```python
from build123d import *

# Parameters (mm, degrees)
EXTRUDE_1_DEPTH          = 3
EXTRUDE_2_DEPTH          = 287
SKETCH_4_W               = 21.736589458
SKETCH_4_H               = 200
CUT_EXTRUDE_1_DEPTH      = 43
SKETCH_5_W               = 23.415155123
SKETCH_5_H               = 200
CUT_EXTRUDE_2_DEPTH      = 43
CUT_EXTRUDE_3_DEPTH      = 259.263552403
HOLE_WIZARD_1_AT_2_COUNT = 2
HOLE_WIZARD_1_AT_2_PITCH = 31.622776602
HOLE_WIZARD_1_AT_3_COUNT = 2
HOLE_WIZARD_1_AT_3_PITCH = 10
HOLE_WIZARD_1_AT_4_COUNT = 2
HOLE_WIZARD_1_AT_4_PITCH = 242.860042
HOLE_WIZARD_1_AT_5_COUNT = 2
HOLE_WIZARD_1_AT_5_PITCH = 241
HOLE_WIZARD_1_AT_6_COUNT = 2
HOLE_WIZARD_1_AT_6_PITCH = 232.939906414
HOLE_WIZARD_1_AT_7_COUNT = 2
HOLE_WIZARD_1_AT_7_PITCH = 231
HOLE_WIZARD_1_AT_8_COUNT = 2
HOLE_WIZARD_1_AT_8_PITCH = 30
SKETCH_10_W              = 190.5
SKETCH_10_H              = 70
CUT_EXTRUDE_4_DEPTH      = 2
SKETCH_11_W              = 190.5
SKETCH_11_H              = 60
CUT_EXTRUDE_5_DEPTH      = 1


with BuildPart() as part:
    # 草图1 → 凸台-拉伸1 (new body)
    with BuildSketch(Plane.XY):
        Polygon((-143.25, 30), (-143.25, 70), (-105.25, 70), (-105.25, 65), (-100.25, 65), (-100.25, 70), (100.75, 70), (100.75, 65), (105.75, 65), (105.75, 70), (143.75, 70), (143.75, 30), (135.75, 30), (135.75, -30), (143.75, -30), (143.75, -70), (105.75, -70), (105.75, -65), (100.75, -65), (100.75, -70), (-100.25, -70), (-100.25, -65), (-105.25, -65), (-105.25, -70), (-143.25, -70), (-143.25, -30), (-135.25, -30), (-135.25, 30), align=None)
    extrude(amount=EXTRUDE_1_DEPTH)

    # 草图2 → 凸台-拉伸2 (add)
    with BuildSketch(Plane.ZY.offset(143.25)):
        with BuildLine():
            Line((0, 70), (0, 30))
            Line((0, 30), (-3, 33))
            Line((-3, 33), (-3, 70))
            ThreePointArc((-3, 70), (6.665476221, 93.334523779), (30, 103))
            Line((30, 103), (47, 103))
            Line((47, 103), (50, 100))
            Line((50, 100), (45, 90))
            Line((45, 90), (60, 90))
            Line((60, 90), (60, 87))
            Line((60, 87), (41, 87))
            Line((41, 87), (47, 100))
            Line((47, 100), (30, 100))
            ThreePointArc((30, 100), (8.786796564, 91.213203436), (0, 70))
        make_face()
        with BuildLine():
            Line((30, -100), (47, -100))
            Line((47, -100), (41, -87))
            Line((41, -87), (60, -87))
            Line((60, -87), (60, -90))
            Line((60, -90), (45, -90))
            Line((45, -90), (50, -100))
            Line((50, -100), (47, -103))
            Line((47, -103), (30, -103))
            ThreePointArc((30, -103), (6.665476221, -93.334523779), (-3, -70))
            Line((-3, -70), (-3, -33))
            Line((-3, -33), (0, -30))
            Line((0, -30), (0, -70))
            ThreePointArc((0, -70), (8.786796564, -91.213203436), (30, -100))
        make_face()
    extrude(amount=-EXTRUDE_2_DEPTH)

    # 草图4 → 切除-拉伸1 (cut)
    with BuildSketch(Plane.ZY.offset(143.25)):
        with Locations((49.368294729, 0)):
            Rectangle(SKETCH_4_W, SKETCH_4_H)
    extrude(amount=-CUT_EXTRUDE_1_DEPTH, mode=Mode.SUBTRACT)

    # 草图5 → 切除-拉伸2 (cut)
    with BuildSketch(Plane(origin=(143.75, 0, 0), x_dir=(0, 0, -1), z_dir=(1, 0, 0))):
        with Locations((-51.459603014, 0)):
            Rectangle(SKETCH_5_W, SKETCH_5_H)
    extrude(amount=-CUT_EXTRUDE_2_DEPTH, mode=Mode.SUBTRACT)

    # 草图6 → 切除-拉伸3 (cut, through all)
    with BuildSketch(Plane(origin=(0, 103, 0), x_dir=(1, 0, 0), z_dir=(0, 1, 0))):
        Polygon((0.25, -30), (-50.25, -30), (-60.25, -50), (-60.25, -55), (59.75, -55), (59.75, -50), (49.75, -30), align=None)
    extrude(amount=-CUT_EXTRUDE_3_DEPTH, mode=Mode.SUBTRACT)

    # 草图9 → 大小六角凹头盖螺钉柱孔1 (revolve, cut)
    with BuildSketch(Plane(origin=(115.75, 15, 0), x_dir=(0, 1, 0), z_dir=(1, 0, 0))):
        Polygon((0, 0), (0, 60), (1.2, 60), (1.2, 2), (2.15, 2), (2.15, 0.024142219), (2.175, 0), align=None)
    hole_wizard_1 = revolve(axis=Axis((115.75, 15, -6.35), (0, 0, 1)), mode=Mode.SUBTRACT)

    # 大小六角凹头盖螺钉柱孔1 at 2: 大小六角凹头盖螺钉柱孔1 ×2
    with Locations(*[Vector(0.3162277660168351, -0.9486832980505148, 0) * (i * HOLE_WIZARD_1_AT_2_PITCH) for i in range(1, HOLE_WIZARD_1_AT_2_COUNT)]):
        add(hole_wizard_1, mode=Mode.SUBTRACT)

    # 大小六角凹头盖螺钉柱孔1 at 3: 大小六角凹头盖螺钉柱孔1 ×2
    with Locations(*[(i * HOLE_WIZARD_1_AT_3_PITCH, 0, 0) for i in range(1, HOLE_WIZARD_1_AT_3_COUNT)]):
        add(hole_wizard_1, mode=Mode.SUBTRACT)

    # 大小六角凹头盖螺钉柱孔1 at 4: 大小六角凹头盖螺钉柱孔1 ×2
    with Locations(*[Vector(-0.9923410949607508, -0.12352793713204367, 0) * (i * HOLE_WIZARD_1_AT_4_PITCH) for i in range(1, HOLE_WIZARD_1_AT_4_COUNT)]):
        add(hole_wizard_1, mode=Mode.SUBTRACT)

    # 大小六角凹头盖螺钉柱孔1 at 5: 大小六角凹头盖螺钉柱孔1 ×2
    with Locations(*[(-i * HOLE_WIZARD_1_AT_5_PITCH, 0, 0) for i in range(1, HOLE_WIZARD_1_AT_5_COUNT)]):
        add(hole_wizard_1, mode=Mode.SUBTRACT)

    # 大小六角凹头盖螺钉柱孔1 at 6: 大小六角凹头盖螺钉柱孔1 ×2
    with Locations(*[Vector(-0.9916720735252418, -0.12878858097730414, 0) * (i * HOLE_WIZARD_1_AT_6_PITCH) for i in range(1, HOLE_WIZARD_1_AT_6_COUNT)]):
        add(hole_wizard_1, mode=Mode.SUBTRACT)

    # 大小六角凹头盖螺钉柱孔1 at 7: 大小六角凹头盖螺钉柱孔1 ×2
    with Locations(*[(-i * HOLE_WIZARD_1_AT_7_PITCH, 0, 0) for i in range(1, HOLE_WIZARD_1_AT_7_COUNT)]):
        add(hole_wizard_1, mode=Mode.SUBTRACT)

    # 大小六角凹头盖螺钉柱孔1 at 8: 大小六角凹头盖螺钉柱孔1 ×2
    with Locations(*[(0, -i * HOLE_WIZARD_1_AT_8_PITCH, 0) for i in range(1, HOLE_WIZARD_1_AT_8_COUNT)]):
        add(hole_wizard_1, mode=Mode.SUBTRACT)

    # 草图10 → 切除-拉伸4 (cut)
    with BuildSketch(Plane.XY.offset(3)):
        Rectangle(SKETCH_10_W, SKETCH_10_H)
    extrude(amount=-CUT_EXTRUDE_4_DEPTH, mode=Mode.SUBTRACT)

    # 草图11 → 切除-拉伸5 (cut)
    with BuildSketch(Plane.XY):
        Rectangle(SKETCH_11_W, SKETCH_11_H)
    extrude(amount=CUT_EXTRUDE_5_DEPTH, mode=Mode.SUBTRACT)


solid = part.part
```
The model under review builds one solid part; all positions refer to its coordinate system, in mm. A direction names the side the tool comes from. Coordinates: 2 decimals unless noted, no trailing zeros. Write each loop counter-clockwise with the first axis right and the second up, starting at its lowest first coordinate (ties: lowest second). Pieces come first, ordered by that corner, then holes. Notation, with made-up numbers: (75.5, 5) - (128.5, 5) arc R24 cw to (128.5, 22) - close; hole circle Ø7 at (25, 32). An arc over 180 degrees is marked (long way). Answer in a Markdown table with one row per item. Add a question column.
Q1. Consider section D-D on z = 15. Give the boundary of the cut face in (x, y), then the cut area to 3 significant figures.
Q2. To check wall thickness, follow line 1 along X through (y, z) = (15, 2.4); line 2 along X through (y, z) = (15, 1.25); line 3 along Y through (x, z) = (-40.5, 28.5). State the ranges of each line that lie inside material, in increasing order. Write a range as from..to.
Q3. Consider section A-A on y = 5. Give the boundary of the cut face in (x, z).
Q4. Clearance check with flat-ended pins moving along their axes: pin 1 (1.5 mm diameter, centred on x = 50, z = 17.5, fed in from +Y); pin 2 (0.9 mm diameter, centred on x = -19.5, y = 88, fed in from -Z); pin 3 (1 mm diameter, centred on x = -29, z = 2.5, fed in from +Y). State where each tip first meets the part, or that it passes through.
Q5. Consider section B-B on z = 36.5. Give the boundary of the cut face in (x, y), then the cut area to 3 significant figures.
Q6. Draft analysis for pull direction Z (two halves, no side actions). For faces 1 (the face through (116, 0, 0)), 2 (the face through (55.93, 100.45, 42.36)), 3 (the face through (100.75, 89, 50)), 4 (the face through (78.696, 95.07, 47.535)), state which applies: +Z half, -Z half, draft (parallel to the pull), parting line (faces both ways), or undercut.
Q7. For faces 5 (the face through (-100.25, 89.7, 48.3)), 6 (the face through (-1.759, 91.445, 9.021)), 7 (the face through (-1, -87, 57)), 8 (the face through (-56.3, 100.4, 42.1)), list the 3-axis set-ups (+Z, -Z, +X, -X, +Y, -Y) from which the entire face can be reached by the end or side of a thin tool; tool diameter is ignored.
Answers below:
| question | item | result |
|---|---|---|
| 1 | outline | (-143.25, -99.39) - (143.75, -99.39) - (143.75, -95.98) - (-143.25, -95.98) - close; (-143.25, 95.98) - (143.75, 95.98) - (143.75, 99.39) - (-143.25, 99.39) - close |
| 1 | area | 1,960 mm² |
| 2 | line 1 | -135.25..-126.45, -124.05..-116.45, -114.05..-95.25, 95.25..114.55, 116.95..124.55, 126.95..135.75 |
| 2 | line 2 | -135.25..-127.4, -123.1..-117.4, -113.1..-95.25, 95.25..113.6, 117.9..123.6, 127.9..135.75 |
| 2 | line 3 | -102.97..-99.96, 99.96..102.97 |
| 3 | outline | (-135.25, 0) - (-95.25, 0) - (-95.25, 3) - (-135.25, 3) - close; (95.25, 0) - (135.75, 0) - (135.75, 3) - (95.25, 3) - close |
| 4 | pin 1 | y = 100.84 |
| 4 | pin 2 | z = 2.05 |
| 4 | pin 3 | y = 88.97 |
| 5 | outline | (-143.25, -103) - (-53.5, -103) - (-53.5, -100) - (-143.25, -100) - close; (-143.25, 100) - (-53.5, 100) - (-53.5, 103) - (-143.25, 103) - close; (53, -103) - (143.75, -103) - (143.75, -100) - (53, -100) - close; (53, 100) - (143.75, 100) - (143.75, 103) - (53, 103) - close |
| 5 | area | 1,080 mm² |
| 6 | face 1 | -Z half |
| 6 | face 2 | undercut |
| 6 | face 3 | draft |
| 6 | face 4 | +Z half |
| 7 | face 5 | +Z, -X |
| 7 | face 6 | +X, -X |
| 7 | face 7 | +Z, +X, -X |
| 7 | face 8 | +Y, -Y |
